Could you check a few things on this model? Use its own coordinates, in mm. A direction names the side the tool comes from. Round coordinates to 2 decimals unless told otherwise and drop trailing zeros. Write each loop counter-clockwise with the first axis right and the second up, starting at its lowest first coordinate (ties: lowest second). Pieces come first, ordered by that corner, then holes. Notation, with made-up numbers: M -28,65.25 L -11,65.25 A21 cw -11,76.25 Z; hole C -28.5,42 d9. An arc over 180 degrees is marked long. One line per item, written item: value. Start each with the question number.
(1) I want a section at A-A on y = -6. Please give me the cut outline in (x, z), and give its area (3 significant figures).
(2) I'm going to push flat-ended pins straight in: pin 1 Ø0.9 at (x, z) = (16.5, 2.5) entering from +Y (3 decimals); pin 2 Ø4 at (y, z) = (-2, 21.5) entering from +X; pin 3 Ø3 at (y, z) = (-4, 32.5) entering from +X. Where does each tip first touch, or does it pass through?
(3) I want a section at B-B on z = 25. Please give me the cut outline in (x, y).
(4) I want a section at C-C on y = -1. Count the separate pieces of the cut face and the enclosed holes in it, and give its area (3 significant figures).
(5) I want a section at D-D on z = 32.5. Please give me the cut outline in (x, y), and give its area (3 significant figures).
(6) Thinking about a two-plate mould opening in X: for faces 4 (the face through (-32.16, 0.74, 2.96)), 5 (the face through (38, -5, 3)), 6 (the face through (-11, -8, 3)), which applies, released by +X, released by -X, zero draft, split by the parting line, or undercut?
(7) Which directions (+Z, -Z, +X, -X, +Y, -Y) give clear straight access to the entire face, cutting with the end or side of a thin tool? Please do faces 1 (the face through (-1, -4, 0)), 2 (the face through (-27, -4, 30)), 3 (the face through (22.404, -0.164, 2.958)).
(8) If I drill on L1, parallel to Z at x = -28.5, y = -5.75; L2, parallel to Z at x = 9, y = -3.25; L3, parallel to X at y = -1.25, z = 26.5, over which ranges is the centre line in solid material (lowest first)?
Solid Edge part; units mm, degrees
sketch "Sketch1" plane through (0, 0, 0) normal (0, 0, 1) x (1, 0, 0)
  line L0 (-38, -8) -> (38, -8)
  line L1 (38, -8) -> (38, -1.875)
  line L2 (38, -1.875) -> (34.7673, -1.875)
  line L3 (34.7673, -1.875) -> (33.5389, 1.5)
  line L4 (33.5389, 1.5) -> (32.4346, 1.5)
  line L5 (32.4346, 1.5) -> (31.2062, -1.875)
  line L6 (31.2062, -1.875) -> (30.0549, -1.875)
  line L7 (30.0549, -1.875) -> (28.8265, 1.5)
  line L8 (28.8265, 1.5) -> (27.7222, 1.5)
  line L9 (27.7222, 1.5) -> (26.4938, -1.875)
  line L10 (26.4938, -1.875) -> (25.3425, -1.875)
  line L11 (25.3425, -1.875) -> (24.1141, 1.5)
  line L12 (24.1141, 1.5) -> (23.0098, 1.5)
  line L13 (23.0098, 1.5) -> (21.7814, -1.875)
  line L14 (21.7814, -1.875) -> (20.6301, -1.875)
  line L15 (20.6301, -1.875) -> (19.4017, 1.5)
  line L16 (19.4017, 1.5) -> (18.2974, 1.5)
  line L17 (18.2974, 1.5) -> (17.069, -1.875)
  line L18 (17.069, -1.875) -> (15.9177, -1.875)
  line L19 (15.9177, -1.875) -> (14.6893, 1.5)
  line L20 (14.6893, 1.5) -> (13.585, 1.5)
  line L21 (13.585, 1.5) -> (12.3566, -1.875)
  line L22 (12.3566, -1.875) -> (11.2053, -1.875)
  line L23 (11.2053, -1.875) -> (9.9769, 1.5)
  line L24 (9.9769, 1.5) -> (8.8726, 1.5)
  line L25 (8.8726, 1.5) -> (7.6442, -1.875)
  line L26 (7.6442, -1.875) -> (6.4929, -1.875)
  line L27 (6.4929, -1.875) -> (5.2645, 1.5)
  line L28 (5.2645, 1.5) -> (4.1602, 1.5)
  line L29 (4.1602, 1.5) -> (2.9318, -1.875)
  line L30 (2.9318, -1.875) -> (1.7805, -1.875)
  line L31 (1.7805, -1.875) -> (0.5521, 1.5)
  line L32 (0.5521, 1.5) -> (-0.5521, 1.5)
  line L33 (-0.5521, 1.5) -> (-1.7805, -1.875)
  line L34 (-1.7805, -1.875) -> (-2.9318, -1.875)
  line L35 (-2.9318, -1.875) -> (-4.1602, 1.5)
  line L36 (-4.1602, 1.5) -> (-5.2645, 1.5)
  line L37 (-5.2645, 1.5) -> (-6.4929, -1.875)
  line L38 (-6.4929, -1.875) -> (-7.6442, -1.875)
  line L39 (-7.6442, -1.875) -> (-8.8726, 1.5)
  line L40 (-8.8726, 1.5) -> (-9.9769, 1.5)
  line L41 (-9.9769, 1.5) -> (-11.2053, -1.875)
  line L42 (-11.2053, -1.875) -> (-12.3566, -1.875)
  line L43 (-12.3566, -1.875) -> (-13.585, 1.5)
  line L44 (-13.585, 1.5) -> (-14.6893, 1.5)
  line L45 (-14.6893, 1.5) -> (-15.9177, -1.875)
  line L46 (-15.9177, -1.875) -> (-17.069, -1.875)
  line L47 (-17.069, -1.875) -> (-18.2974, 1.5)
  line L48 (-18.2974, 1.5) -> (-19.4017, 1.5)
  line L49 (-19.4017, 1.5) -> (-20.6301, -1.875)
  line L50 (-20.6301, -1.875) -> (-21.7814, -1.875)
  line L51 (-21.7814, -1.875) -> (-23.0098, 1.5)
  line L52 (-23.0098, 1.5) -> (-24.1141, 1.5)
  line L53 (-24.1141, 1.5) -> (-25.3425, -1.875)
  line L54 (-25.3425, -1.875) -> (-26.4938, -1.875)
  line L55 (-26.4938, -1.875) -> (-27.7222, 1.5)
  line L56 (-27.7222, 1.5) -> (-28.8265, 1.5)
  line L57 (-28.8265, 1.5) -> (-30.0549, -1.875)
  line L58 (-30.0549, -1.875) -> (-31.2062, -1.875)
  line L59 (-31.2062, -1.875) -> (-32.4346, 1.5)
  line L60 (-32.4346, 1.5) -> (-33.5389, 1.5)
  line L61 (-33.5389, 1.5) -> (-34.7673, -1.875)
  line L62 (-34.7673, -1.875) -> (-38, -1.875)
  line L63 (-38, -1.875) -> (-38, -8)
extrude "Protrusion1" add sketch "Sketch1" along normal blind 6
sketch "Sketch2" plane through (0, 0, 0) normal (0, 0, 1) x (1, 0, 0)
  line L0 (-38, -8) -> (-30, -8)
  line L1 (-30, -8) -> (-30, 0)
  line L2 (-30, 0) -> (-38, 0)
  line L3 (-38, 0) -> (-38, -8)
extrude "ExtrudedProtrusion_2" add sketch "Sketch2" along normal blind 36
sketch "Sketch3" plane through (0, 0, 30) normal (0, 0, 1) x (1, 0, 0)
  line L0 (-38, -8) -> (-24, -8)
  line L1 (-24, -8) -> (-24, 0)
  line L2 (-24, 0) -> (-38, 0)
  line L3 (-38, 0) -> (-38, -8)
extrude "ExtrudedProtrusion_3" add sketch "Sketch3" along normal blind 6
Found:
1. outline: M -38,0 L 38,0 L 38,6 L -30,6 L -30,30 L -24,30 L -24,36 L -38,36 Z
1. area: 732 mm²
2. pin 1: stops at y = -1.875
2. pin 2: stops at x = -30
2. pin 3: stops at x = -24
3. outline: M -38,-8 L -30,-8 L -30,0 L -38,0 Z
4. separate pieces: 15
4. enclosed holes: 0
4. area: 570 mm²
5. outline: M -38,-8 L -24,-8 L -24,0 L -38,0 Z
5. area: 112 mm²
6. face 4: undercut
6. face 5: released by +X
6. face 6: zero draft
7. face 1: -Z, +X, -X, +Y, -Y
7. face 2: +X, +Y, -Y
7. face 3: +Z, -Z, +Y
8. L1: z = 0 to 6, 30 to 36
8. L2: z = 0 to 6
8. L3: x = -38 to -30
